```python
from build123d import *

# Parameters (mm, degrees)
BOSS_EXTRUDE1_DEPTH = 10


with BuildPart() as part:
    # Sketch1 → Boss-Extrude1 (new body)
    with BuildSketch(Plane.XY):
        with BuildLine():
            ThreePointArc((10.996962206, -0.2585), (11, 0), (10.996962206, 0.2585))
            ThreePointArc((10.996962206, 0.2585), (9.901430175, 0.801787583), (8.692954638, 0.988706562))
            ThreePointArc((8.692954638, 0.988706562), (8.641285292, 1.368645135), (8.573018284, 1.745954896))
            ThreePointArc((8.573018284, 1.745954896), (9.664585678, 2.297164887), (10.538613458, 3.152400099))
            ThreePointArc((10.538613458, 3.152400099), (10.461621679, 3.399186938), (10.378851672, 3.644096317))
            ThreePointArc((10.378851672, 3.644096317), (9.169053699, 3.822255499), (7.961964024, 3.626586533))
            ThreePointArc((7.961964024, 3.626586533), (7.79541608, 3.971962882), (7.613895169, 4.309710124))
            ThreePointArc((7.613895169, 4.309710124), (8.481704197, 5.171254853), (9.048671798, 6.254721311))
            ThreePointArc((9.048671798, 6.254721311), (8.899186938, 6.465637775), (8.744786823, 6.672983097))
            ThreePointArc((8.744786823, 6.672983097), (7.539146363, 6.468574414), (6.451600897, 5.909470946))
            ThreePointArc((6.451600897, 5.909470946), (6.186477229, 6.186477229), (5.909470946, 6.451600897))
            ThreePointArc((5.909470946, 6.451600897), (6.468574414, 7.539146363), (6.672983097, 8.744786823))
            ThreePointArc((6.672983097, 8.744786823), (6.465637775, 8.899186938), (6.254721311, 9.048671798))
            ThreePointArc((6.254721311, 9.048671798), (5.171254853, 8.481704197), (4.309710124, 7.613895169))
            ThreePointArc((4.309710124, 7.613895169), (3.971962882, 7.79541608), (3.626586533, 7.961964024))
            ThreePointArc((3.626586533, 7.961964024), (3.822255499, 9.169053699), (3.644096317, 10.378851672))
            ThreePointArc((3.644096317, 10.378851672), (3.399186938, 10.461621679), (3.152400099, 10.538613458))
            ThreePointArc((3.152400099, 10.538613458), (2.297164887, 9.664585678), (1.745954896, 8.573018284))
            ThreePointArc((1.745954896, 8.573018284), (1.368645135, 8.641285292), (0.988706562, 8.692954638))
            ThreePointArc((0.988706562, 8.692954638), (0.801787583, 9.901430175), (0.2585, 10.996962206))
            ThreePointArc((0.2585, 10.996962206), (0, 11), (-0.2585, 10.996962206))
            ThreePointArc((-0.2585, 10.996962206), (-0.801787583, 9.901430175), (-0.988706562, 8.692954638))
            ThreePointArc((-0.988706562, 8.692954638), (-1.368645135, 8.641285292), (-1.745954896, 8.573018284))
            ThreePointArc((-1.745954896, 8.573018284), (-2.297164887, 9.664585678), (-3.152400099, 10.538613458))
            ThreePointArc((-3.152400099, 10.538613458), (-3.399186938, 10.461621679), (-3.644096317, 10.378851672))
            ThreePointArc((-3.644096317, 10.378851672), (-3.822255499, 9.169053699), (-3.626586533, 7.961964024))
            ThreePointArc((-3.626586533, 7.961964024), (-3.971962882, 7.79541608), (-4.309710124, 7.613895169))
            ThreePointArc((-4.309710124, 7.613895169), (-5.171254853, 8.481704197), (-6.254721311, 9.048671798))
            ThreePointArc((-6.254721311, 9.048671798), (-6.465637775, 8.899186938), (-6.672983097, 8.744786823))
            ThreePointArc((-6.672983097, 8.744786823), (-6.468574414, 7.539146363), (-5.909470946, 6.451600897))
            ThreePointArc((-5.909470946, 6.451600897), (-6.186477229, 6.186477229), (-6.451600897, 5.909470946))
            ThreePointArc((-6.451600897, 5.909470946), (-7.539146363, 6.468574414), (-8.744786823, 6.672983097))
            ThreePointArc((-8.744786823, 6.672983097), (-8.899186938, 6.465637775), (-9.048671798, 6.254721311))
            ThreePointArc((-9.048671798, 6.254721311), (-8.481704197, 5.171254853), (-7.613895169, 4.309710124))
            ThreePointArc((-7.613895169, 4.309710124), (-7.79541608, 3.971962882), (-7.961964024, 3.626586533))
            ThreePointArc((-7.961964024, 3.626586533), (-9.169053699, 3.822255499), (-10.378851672, 3.644096317))
            ThreePointArc((-10.378851672, 3.644096317), (-10.461621679, 3.399186938), (-10.538613458, 3.152400099))
            ThreePointArc((-10.538613458, 3.152400099), (-9.664585678, 2.297164887), (-8.573018284, 1.745954896))
            ThreePointArc((-8.573018284, 1.745954896), (-8.641285292, 1.368645135), (-8.692954638, 0.988706562))
            ThreePointArc((-8.692954638, 0.988706562), (-9.901430175, 0.801787583), (-10.996962206, 0.2585))
            ThreePointArc((-10.996962206, 0.2585), (-11, 0), (-10.996962206, -0.2585))
            ThreePointArc((-10.996962206, -0.2585), (-9.901430175, -0.801787583), (-8.692954638, -0.988706562))
            ThreePointArc((-8.692954638, -0.988706562), (-8.641285292, -1.368645135), (-8.573018284, -1.745954896))
            ThreePointArc((-8.573018284, -1.745954896), (-9.664585678, -2.297164887), (-10.538613458, -3.152400099))
            ThreePointArc((-10.538613458, -3.152400099), (-10.461621679, -3.399186938), (-10.378851672, -3.644096317))
            ThreePointArc((-10.378851672, -3.644096317), (-9.169053699, -3.822255499), (-7.961964024, -3.626586533))
            ThreePointArc((-7.961964024, -3.626586533), (-7.79541608, -3.971962882), (-7.613895169, -4.309710124))
            ThreePointArc((-7.613895169, -4.309710124), (-8.481704197, -5.171254853), (-9.048671798, -6.254721311))
            ThreePointArc((-9.048671798, -6.254721311), (-8.899186938, -6.465637775), (-8.744786823, -6.672983097))
            ThreePointArc((-8.744786823, -6.672983097), (-7.539146363, -6.468574414), (-6.451600897, -5.909470946))
            ThreePointArc((-6.451600897, -5.909470946), (-6.186477229, -6.186477229), (-5.909470946, -6.451600897))
            ThreePointArc((-5.909470946, -6.451600897), (-6.468574414, -7.539146363), (-6.672983097, -8.744786823))
            ThreePointArc((-6.672983097, -8.744786823), (-6.465637775, -8.899186938), (-6.254721311, -9.048671798))
            ThreePointArc((-6.254721311, -9.048671798), (-5.171254853, -8.481704197), (-4.309710124, -7.613895169))
            ThreePointArc((-4.309710124, -7.613895169), (-3.971962882, -7.79541608), (-3.626586533, -7.961964024))
            ThreePointArc((-3.626586533, -7.961964024), (-3.822255499, -9.169053699), (-3.644096317, -10.378851672))
            ThreePointArc((-3.644096317, -10.378851672), (-3.399186938, -10.461621679), (-3.152400099, -10.538613458))
            ThreePointArc((-3.152400099, -10.538613458), (-2.297164887, -9.664585678), (-1.745954896, -8.573018284))
            ThreePointArc((-1.745954896, -8.573018284), (-1.368645135, -8.641285292), (-0.988706562, -8.692954638))
            ThreePointArc((-0.988706562, -8.692954638), (-0.801787583, -9.901430175), (-0.2585, -10.996962206))
            ThreePointArc((-0.2585, -10.996962206), (0, -11), (0.2585, -10.996962206))
            ThreePointArc((0.2585, -10.996962206), (0.801787583, -9.901430175), (0.988706562, -8.692954638))
            ThreePointArc((0.988706562, -8.692954638), (1.368645135, -8.641285292), (1.745954896, -8.573018284))
            ThreePointArc((1.745954896, -8.573018284), (2.297164887, -9.664585678), (3.152400099, -10.538613458))
            ThreePointArc((3.152400099, -10.538613458), (3.399186938, -10.461621679), (3.644096317, -10.378851672))
            ThreePointArc((3.644096317, -10.378851672), (3.822255499, -9.169053699), (3.626586533, -7.961964024))
            ThreePointArc((3.626586533, -7.961964024), (3.971962882, -7.79541608), (4.309710124, -7.613895169))
            ThreePointArc((4.309710124, -7.613895169), (5.171254853, -8.481704197), (6.254721311, -9.048671798))
            ThreePointArc((6.254721311, -9.048671798), (6.465637775, -8.899186938), (6.672983097, -8.744786823))
            ThreePointArc((6.672983097, -8.744786823), (6.468574414, -7.539146363), (5.909470946, -6.451600897))
            ThreePointArc((5.909470946, -6.451600897), (6.186477229, -6.186477229), (6.451600897, -5.909470946))
            ThreePointArc((6.451600897, -5.909470946), (7.539146363, -6.468574414), (8.744786823, -6.672983097))
            ThreePointArc((8.744786823, -6.672983097), (8.899186938, -6.465637775), (9.048671798, -6.254721311))
            ThreePointArc((9.048671798, -6.254721311), (8.481704197, -5.171254853), (7.613895169, -4.309710124))
            ThreePointArc((7.613895169, -4.309710124), (7.79541608, -3.971962882), (7.961964024, -3.626586533))
            ThreePointArc((7.961964024, -3.626586533), (9.169053699, -3.822255499), (10.378851672, -3.644096317))
            ThreePointArc((10.378851672, -3.644096317), (10.461621679, -3.399186938), (10.538613458, -3.152400099))
            ThreePointArc((10.538613458, -3.152400099), (9.664585678, -2.297164887), (8.573018284, -1.745954896))
            ThreePointArc((8.573018284, -1.745954896), (8.641285292, -1.368645135), (8.692954638, -0.988706562))
            ThreePointArc((8.692954638, -0.988706562), (9.901430175, -0.801787583), (10.996962206, -0.2585))
        make_face()
        with BuildLine():
            Line((-2.24374247, 2.35), (2.24374247, 2.35))
            ThreePointArc((2.24374247, 2.35), (3.15, 0), (2.24374247, -2.35))
            Line((2.24374247, -2.35), (-2.24374247, -2.35))
            ThreePointArc((-2.24374247, -2.35), (-3.15, 0), (-2.24374247, 2.35))
        make_face(mode=Mode.SUBTRACT)
    extrude(amount=BOSS_EXTRUDE1_DEPTH)


solid = part.part
```
Check sheet for the modelled part. Datum: model origin and axes. Units: mm. A direction names the side the tool comes from. Round coordinates to 2 decimals unless told otherwise and drop trailing zeros. Write each loop counter-clockwise with the first axis right and the second up, starting at its lowest first coordinate (ties: lowest second). Pieces come first, ordered by that corner, then holes. Notation, with made-up numbers: (60, 36.5) -> (68, 36.5) arc R7 cw to (68, 42.5) -> close; hole circle Ø9 at (-30, 16). An arc over 180 degrees is marked (long way). One line per question, with ' | ' between items. Start each with the question number.
1. Sectioned sample at D-D, the plane y = 7.25. Record the cut outline in (x, z).
2. Sectioned sample at B-B, the plane x = 9.5. Record the cut outline in (y, z), then the cut area to 3 significant figures.
3. Sectioned sample at C-C, the plane x = -2.75. Record the cut outline in (y, z), then the cut area to 3 significant figures.
4. Release check for a two-part mould opening along Y. For faces 1 (the face through (2.287, -9.651, 4.93)), 2 (the face through (6.463, 7.523, 4.93)), 3 (the face through (9.186, 3.822, 4.93)), 4 (the face through (-2.287, 9.651, 4.93)) record: +Y half, -Y half, draft (parallel to the pull), parting line (faces both ways), or undercut.
5. Sectioned sample at A-A, the plane y = 9.75. Record the cut outline in (x, z).
6. Depth check by flat-ended pin: pin 1 (1.5 mm diameter, centred on y = 4, z = 5.5, fed in from -X); pin 2 (1.5 mm diameter, centred on x = 8, z = 2.5, fed in from -Y); pin 3 (3 mm diameter, centred on y = 7, z = 8, fed in from +X). Enter the tip coordinate at first touch or a pass-through.
7. Set-up check for faces 5 (the face through (-9.651, -2.287, 4.93)), 6 (the face through (-0.797, 9.918, 4.93)), 7 (the face through (3.15, 0.04, 4.93)): record each of +Z, -Z, +X, -X, +Y, -Y from which the full face is reachable in a straight line by a thin tool's end or side.
8. Scan lines: line 1 along X through (y, z) = (9.5, 8.5); line 2 along Y through (x, z) = (6, 1); line 3 along Y through (x, z) = (-9.25, 5.5). Record each from-to range of solid material in increasing order. Write a range as from..to.
Taken from the geometry:
1) outline: (-6.36, 0) -> (6.36, 0) -> (6.36, 10) -> (-6.36, 10) -> close
2) outline: (-3.81, 0) -> (-2.19, 0) -> (-2.19, 10) -> (-3.81, 10) -> close; (-0.91, 0) -> (0.91, 0) -> (0.91, 10) -> (-0.91, 10) -> close; (2.19, 0) -> (3.81, 0) -> (3.81, 10) -> (2.19, 10) -> close | area: 50.6 mm^2
3) outline: (-10.19, 0) -> (-1.62, 0) -> (-1.62, 10) -> (-10.19, 10) -> close; (1.62, 0) -> (10.19, 0) -> (10.19, 10) -> (1.62, 10) -> close | area: 171 mm^2
4) face 1: -Y half | face 2: undercut | face 3: undercut | face 4: +Y half
5) outline: (-3.78, 0) -> (-2.36, 0) -> (-2.36, 10) -> (-3.78, 10) -> close; (-0.85, 0) -> (0.85, 0) -> (0.85, 10) -> (-0.85, 10) -> close; (2.36, 0) -> (3.78, 0) -> (3.78, 10) -> (2.36, 10) -> close
6) pin 1: stops at x = -10.51 | pin 2: stops at y = -6.67 | pin 3: stops at x = 9.05
7) face 5: +Z, -Z, -X | face 6: +Z, -Z, +Y | face 7: +Z, -Z
8) line 1: x = -3.81..-2.19, -0.91..0.91, 2.19..3.81 | line 2: y = -8.95..-6.58, -6.37..6.37, 6.58..8.95 | line 3: y = -3.82..-2.04, -0.95..0.95, 2.04..3.82
